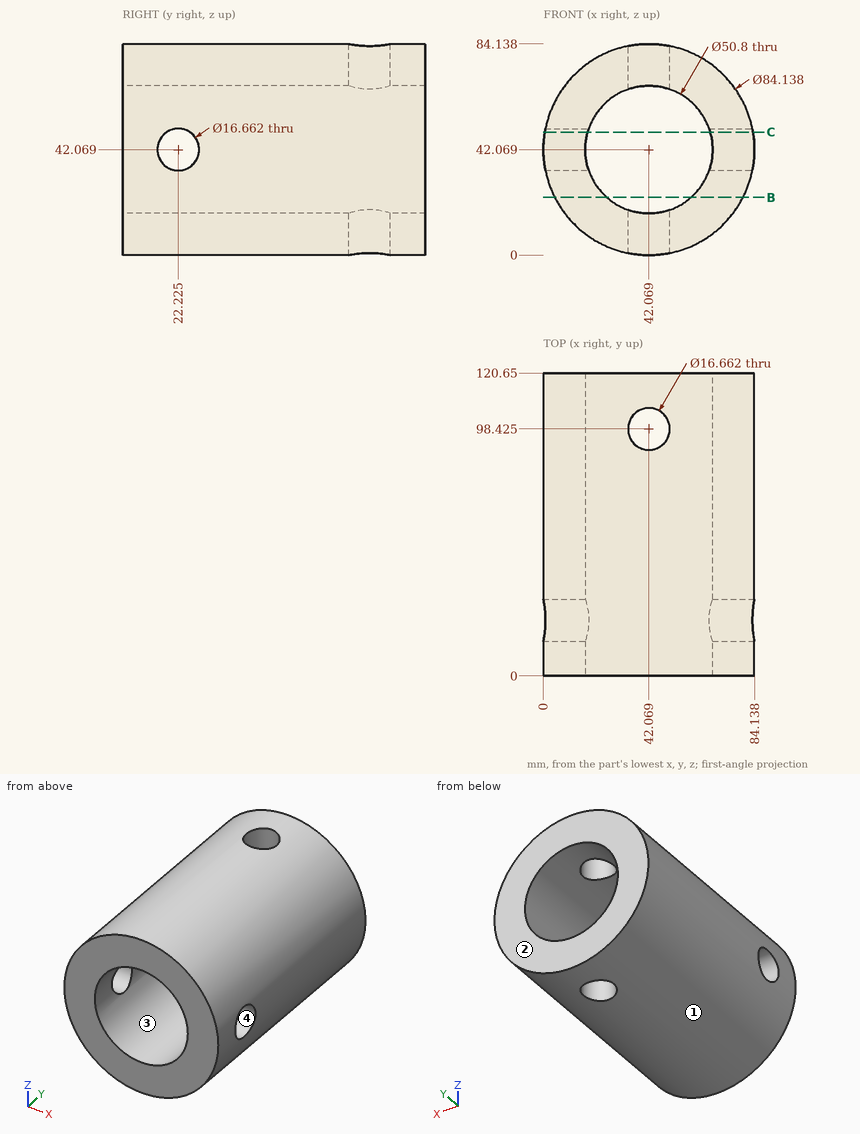
Part print with two shaded views. Sizes in mm from the minimum x, y, z corner. Coordinates: 2 decimals unless noted, no trailing zeros. Write each loop counter-clockwise with the first axis right and the second up, starting at its lowest first coordinate (ties: lowest second). Pieces come first, ordered by that corner, then holes. Notation, with made-up numbers: (-25, 54) - (3, 54) arc R19 ccw to (3, 65) - close; hole circle Ø5 at (40.5, 69). An arc over 180 degrees is marked (long way). Put each result on its own line as item: value.
1. Band-saw the part on B-B (z = 23). Write the cut outline in (x, y), then the cut area to 3 significant figures.
Final values:
outline: (4.57, 0) - (25.29, 0) - (25.29, 120.65) - (4.57, 120.65) - close; (58.85, 0) - (79.57, 0) - (79.57, 120.65) - (58.85, 120.65) - close
area: 5,000 mm²
2. Band-saw the part on C-C (z = 49). Give the number of separate pieces and of enclosed holes in the cut face, then the cut area to 3 significant figures.
Final values:
separate pieces: 4
enclosed holes: 0
area: 3,800 mm²
3. Probe line 1 along Z through (x, y) = (42, 41); line 2 along Z through (x, y) = (47.5, 89.5) (1 decimal); line 3 along X through (y, z) = (6, 7.5) (1 decimal). List the from-to ranges inside material, lowest first. Write a range as [from, to].
Final values:
line 1: z = [0, 16.67], [67.47, 84.14]
line 2: z = [0.4, 17.3], [66.9, 83.8]
line 3: x = [18.1, 66]
4. Flat gauge pins, fed straight in: pin 1 Ø1 at (x, y) = (17.5, 51) entering from +Z; pin 2 Ø2 at (y, z) = (24.5, 24.5) entering from -X; pin 3 Ø5 at (y, z) = (63, 46) entering from +X. Where does each tip first touch, or does it go through?
Final values:
pin 1: stops at z = 76.57
pin 2: stops at x = 3.4
pin 3: stops at x = 84.11
5. Two-plate mould, pull along Z, no slides. Class the marked faces 1, 2, 3 and 4: +Z half, -Z half, draft (parallel to the pull), parting line (faces both ways), or undercut.
Final values:
face 1: parting line
face 2: draft
face 3: undercut
face 4: undercut
